Geometry: final body of the model. Coordinates: model frame, mm. Face numbers are marked on the shaded views. A direction names the side the tool comes from. Round coordinates to 2 decimals unless told otherwise and drop trailing zeros. Write each loop counter-clockwise with the first axis right and the second up, starting at its lowest first coordinate (ties: lowest second). Pieces come first, ordered by that corner, then holes. Notation, with made-up numbers: (-34, -37.5) - (12, -37.5) arc R12 ccw to (12, -33.5) - close; hole circle Ø3 at (-24, 69). An arc over 180 degrees is marked (long way). Write each question's results on one line, items separated by ' | '.
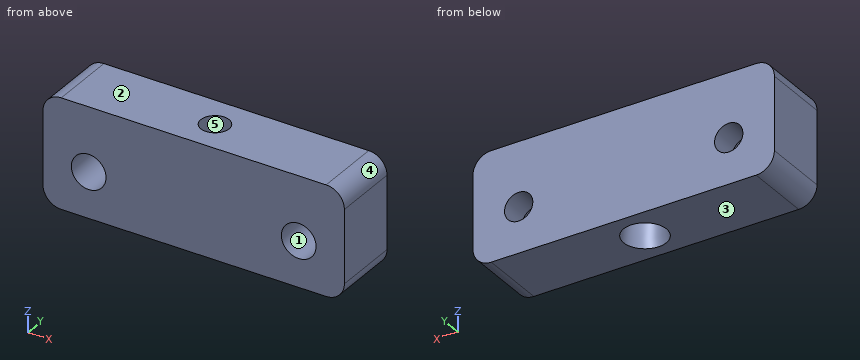
from build123d import *

# Parameters (mm, degrees)
ESQUISSE1_W             = 33
ESQUISSE1_H             = 12
ESQUISSE1_R             = 1.55
BOSS_EXTRU_1_DEPTH      = 3.65
ENL_V_START             = -3
ESQUISSE5_R             = 1.9
ENL_V_MAT_EXTRU_3_DEPTH = 19.668871683
CONG_1_R                = 2


with BuildPart() as part:
    # Esquisse1 → Boss.-Extru.1 (new, symmetric)
    with BuildSketch(Plane(origin=(0, 0, 0), x_dir=(1, 0, 0), z_dir=(0, 1, 0))):
        with Locations((0, 6)):
            Rectangle(ESQUISSE1_W, ESQUISSE1_H)
        with Locations(Location((-11.5, 7, 0), (0, 0, 270))):
            Circle(ESQUISSE1_R, mode=Mode.SUBTRACT)
        with Locations(Location((11.5, 7, 0), (0, 0, 90))):
            Circle(ESQUISSE1_R, mode=Mode.SUBTRACT)
    extrude(amount=BOSS_EXTRU_1_DEPTH, both=True)

    # Esquisse4 → Enlèvement de matière-Révolution1 (revolve, cut)
    with BuildSketch(Plane(origin=(0, 0, 0), x_dir=(0, 0, -1), z_dir=(1, 0, 0)), mode=Mode.PRIVATE) as enl_vement_de_mati_re_r_volution1_sk:
        Polygon((0, 0), (12, 0), (12, 2.337443318), (7, 1.9), (3, 1.9), (3, 1.55), (0, 1.55), align=None)
    revolve(enl_vement_de_mati_re_r_volution1_sk.sketch.rotate(Axis((0, 0, 12), (0, 0, -1)), 90), axis=Axis((0, 0, 12), (0, 0, -1)), mode=Mode.SUBTRACT)

    # Esquisse5 → Enlèv. mat.-Extru.3 (cut, through all)
    with BuildSketch(Plane(origin=(0, 3.65, 0), x_dir=(1, 0, 0), z_dir=(0, 1, 0)).offset(ENL_V_START)):
        with Locations(Location((-11.5, 7, 0), (0, 0, 270))):
            Circle(ESQUISSE5_R)
        with Locations(Location((11.5, 7, 0), (0, 0, 270))):
            Circle(ESQUISSE5_R)
    extrude(amount=-ENL_V_MAT_EXTRU_3_DEPTH, mode=Mode.SUBTRACT)

    # Congé1
    cong_1_edges = [part.edges().sort_by_distance(p)[0] for p in [
        (-16.5, 0, -12),
        (16.5, 0, -12),
        (16.5, 0, 0),
        (-16.5, 0, 0),
    ]]
    fillet(cong_1_edges, radius=CONG_1_R)


solid = part.part
Q1. Pin query (flat end, axial travel): pin 1 (1.9 mm diameter, centred on x = -11, z = -6.5, fed in from -Y); pin 2 (3 mm diameter, centred on x = 11.5, z = -7, fed in from +Y); pin 3 (1.9 mm diameter, centred on x = 0.5, y = -0.5, fed in from -Z). Return the tip coordinate at first contact, or that it passes through.
Answer block:
pin 1: y = 0.65 | pin 2: through | pin 3: z = -3
Q2. Section query A-A, the plane x = -11.5. Return loops of the section in (y, z).
Answer block:
outline: (-3.65, -12) - (3.65, -12) - (3.65, -8.55) - (0.65, -8.55) - (0.65, -8.9) - (-3.65, -8.9) - close; (-3.65, -5.1) - (0.65, -5.1) - (0.65, -5.45) - (3.65, -5.45) - (3.65, 0) - (-3.65, 0) - close
Q3. Section query B-B, the plane z = -8. Return loops of the section in (x, y), plus the area to 3 significant figures.
Answer block:
outline: (-16.5, -3.65) - (-13.12, -3.65) - (-13.12, 0.65) - (-12.68, 0.65) - (-12.68, 3.65) - (-16.5, 3.65) - close; (-10.32, 0.65) - (-9.88, 0.65) - (-9.88, -3.65) - (9.88, -3.65) - (9.88, 0.65) - (10.32, 0.65) - (10.32, 3.65) - (-10.32, 3.65) - close; (12.68, 0.65) - (13.12, 0.65) - (13.12, -3.65) - (16.5, -3.65) - (16.5, 3.65) - (12.68, 3.65) - close; hole circle Ø3.97 at (0, 0) | area: 186 mm2
Q4. Access query for the marked faces 1 and 2. Directions: +Z, -Z, +X, -X, +Y, -Y. A direction counts if a zero-diameter tool reaches every point of the face in a straight line with its end or side. Return the directions, or none.
Answer block:
face 1: -Y | face 2: +Z, +X, -X, +Y, -Y
Q5. Section query C-C, the plane z = -2.5. Return loops of the section in (x, y).
Answer block:
outline: (-16.5, -3.65) - (16.5, -3.65) - (16.5, 3.65) - (-16.5, 3.65) - close; hole circle Ø3.1 at (0, 0)
Q6. Section query D-D, the plane y = -1.25. Give the number of separate pieces and of enclosed holes in the cut face, plus the area to 3 significant figures.
Answer block:
separate pieces: 2 | enclosed holes: 2 | area: 336 mm2
Q7. Mould query, pull axis X, two halves, no side actions, for the marked faces 3, 4 and 5. Classes: pulls with the +X half, pulls with the -X half, needs draft (parallel to the pull), parting line crosses it, or undercut.
Answer block:
face 3: needs draft | face 4: pulls with the +X half | face 5: undercut
Q8. Ray query, line 1 along X through (y, z) = (-2.25, -7); line 2 along X through (y, z) = (2.3, -7); line 3 along Z through (x, y) = (-11.5, 1.35). Return the intervals inside material, ascending.
Answer block:
line 1: -16.5 to -13.4, -9.6 to 9.6, 13.4 to 16.5 | line 2: -16.5 to -13.05, -9.95 to 9.95, 13.05 to 16.5 | line 3: -12 to -8.55, -5.45 to 0
